from build123d import *

# Parameters (mm, degrees)
F1_DEPTH = 40
F2_DEPTH = 40
F3_DEPTH = 17


with BuildPart() as f1:
    # F0 (on Front) → F1 (new body)
    with BuildSketch(Plane.XZ):
        with BuildLine():
            ThreePointArc((21.92031, 12.020815), (24.217842, 6.204524), (25, 0))
            ThreePointArc((25, 0), (-21.511862, -12.737339), (12.020815, 21.92031))
            Line((12.020815, 21.92031), (12.388793, 22.288288))
            ThreePointArc((12.388793, 22.288288), (-21.979129, -12.929342), (25.5, 0))
            ThreePointArc((25.5, 0), (24.684017, 6.399166), (22.288288, 12.388793))
            Line((22.288288, 12.388793), (21.92031, 12.020815))
        make_face()
    extrude(amount=-F1_DEPTH)

    # F0 (on Front) → F2 (join)
    with BuildSketch(Plane.XZ):
        with BuildLine():
            ThreePointArc((12.020815, 21.92031), (17.67767, 17.67767), (21.92031, 12.020815))
            Line((21.92031, 12.020815), (22.288288, 12.388793))
            ThreePointArc((22.288288, 12.388793), (18.031223, 18.031223), (12.388793, 22.288288))
            Line((12.388793, 22.288288), (12.020815, 21.92031))
        make_face()
    extrude(amount=-F2_DEPTH)

    # F0 (on Front) → F3 (cut)
    with BuildSketch(Plane.XZ):
        with BuildLine():
            ThreePointArc((12.020815, 21.92031), (17.67767, 17.67767), (21.92031, 12.020815))
            Line((21.92031, 12.020815), (22.288288, 12.388793))
            ThreePointArc((22.288288, 12.388793), (18.031223, 18.031223), (12.388793, 22.288288))
            Line((12.388793, 22.288288), (12.020815, 21.92031))
        make_face()
    extrude(amount=-F3_DEPTH, mode=Mode.SUBTRACT)


solid = f1.part
Here's how the part is built. I have some questions about the finished solid (model axes, mm). Give positions to 0.01 mm unless a question says otherwise; leave off trailing zeros. Loops run counter-clockwise (first coordinate to the right, second up) from the corner with the lowest first, then second, coordinate; pieces in that order, holes last. Notation, with made-up numbers: (75, 64.5) -> (110, 64.5) arc R13 cw to (110, 86.5) -> close; hole circle Ø2 at (2.25, -13). An arc over 180 degrees is marked (long way). Answer as a JSON object with one key per item and string values. Group by question number.
Item 1: Imagine slicing it at A-A on x = 0. Write out the boundary of the cut face in (y, z).
Item 2: Imagine slicing it at D-D on y = 11.5. Write out the boundary of the cut face in (x, z), then the cut area to 3 significant figures.
Item 3: Thinking about a two-plate mould opening in Z: for faces 1 (the cylindrical face through (-22.437, 19.72, -12.118)), 2 (the flat face through (11.21, 0, -22.55)), 3 (the cylindrical face through (17.607, 28.339, 17.748)), which applies, pulls with the +Z half, pulls with the -Z half, needs draft (parallel to the pull), parting line crosses it, or undercut?
Item 4: Will these pins go through, and if not, where does the flat tip stop? pin 1 (5 mm diameter, centred on x = -8.5, y = 18, fed in from -Z); pin 2 (5 mm diameter, centred on x = -3.5, y = 33, fed in from -Z); pin 3 (5 mm diameter, centred on x = 17.5, z = 18.5, fed in from -Y).
Item 5: Imagine slicing it at C-C on y = 29.5. Write out the boundary of the cut face in (x, z).
Item 6: I need wall thicknesses on L1, parallel to Z at x = 0, y = 25; L2, parallel to X at y = 20, z = 0.5 (3 decimals); L3, parallel to Z at x = 9, y = 25. Which ranges of each line are inside material? Lowest first, please.
Item 7: Imagine slicing it at B-B on z = -16.5. Write out the boundary of the cut face in (x, y).
Answer list:
{
 "1": {"outline": "(0, -25.5) -> (40, -25.5) -> (40, -25) -> (0, -25) -> close; (0, 25) -> (40, 25) -> (40, 25.5) -> (0, 25.5) -> close"},
 "2": {"outline": "(12.02, 21.92) -> (12.39, 22.29) arc R25.5 ccw (long way) to (25.5, 0) arc R25.5 ccw to (22.29, 12.39) -> (21.92, 12.02) arc R25 cw to (25, 0) arc R25 cw (long way) to start", "area": "72.2 mm2"},
 "3": {"face 1": "parting line crosses it", "face 2": "needs draft", "face 3": "undercut"},
 "4": {"pin 1": "stops at z = -24.78", "pin 2": "stops at z = -25.48", "pin 3": "stops at y = 17"},
 "5": {"outline": "(12.39, 22.29) arc R25.5 ccw (long way) to (25.5, 0) arc R25.5 ccw to (22.29, 12.39) arc R25.5 ccw to start; hole (12.02, 21.92) arc R25 ccw (long way) to (25, 0) arc R25 ccw to (21.92, 12.02) arc R25 ccw to start"},
 "6": {"L1": "z = -25.5 to -25, 25 to 25.5", "L2": "x = -25.495 to -24.995, 24.995 to 25.495", "L3": "z = -23.86 to -23.32, 23.32 to 23.86"},
 "7": {"outline": "(-19.44, 0) -> (-18.78, 0) -> (-18.78, 40) -> (-19.44, 40) -> close; (18.78, 0) -> (19.44, 0) -> (19.44, 40) -> (18.78, 40) -> close"}
}
